from build123d import *

# Parameters (mm, degrees)
BASPROSKE_W             = 3.175
BASPROSKE_H             = 6.35
TOOTHCUT_DEPTH          = 10.525
TEETHCUTS_COUNT         = 10
TEETHCUTS_ANGLE         = 324
BORSKE_R                = 0.99949
BORE_DEPTH              = 50.8000508
SKETCH1_W               = 3.937
SKETCH1_H               = 3.937
CUT_EXTRUDE1_DEPTH      = 10.344170464
CUT_EXTRUDE1_DEPTH_BACK = 10.344170464


with BuildPart() as part:
    # BasProSke → Base-Revolve (revolve)
    with BuildSketch(Plane(origin=(0, 0, 0), x_dir=(1, 0, 0), z_dir=(0, 1, 0)), mode=Mode.PRIVATE) as base_revolve_sk:
        with Locations((1.5875, 3.175)):
            Rectangle(BASPROSKE_W, BASPROSKE_H)
    revolve(base_revolve_sk.sketch.rotate(Axis((-10, 0, 0), (1, 0, 0)), 180), axis=Axis((-10, 0, 0), (1, 0, 0)))

    # TooCutSke → ToothCut (cut, through all)
    with BuildSketch(Plane(origin=(0, 0, 0), x_dir=(0, 0, -1), z_dir=(1, 0, 0))):
        with BuildLine():
            ThreePointArc((0.630210727, 3.920537785), (0, 3.970866667), (-0.630210727, 3.920537785))
            ThreePointArc((-0.630210727, 3.920537785), (-0.900510691, 5.2110639), (-1.88228345, 6.091201374))
            ThreePointArc((-1.88228345, 6.091201374), (0, 6.3754), (1.88228345, 6.091201374))
            ThreePointArc((1.88228345, 6.091201374), (0.900510691, 5.2110639), (0.630210727, 3.920537785))
        make_face()
    toothcut = extrude(amount=TOOTHCUT_DEPTH, mode=Mode.SUBTRACT)

    # TeethCuts: ToothCut ×10 about axis
    teethcuts_axis = Axis((-10, 0, 0), (1, 0, 0))
    for i in range(1, TEETHCUTS_COUNT):
        add(toothcut.rotate(teethcuts_axis, i * TEETHCUTS_ANGLE / (TEETHCUTS_COUNT - 1)), mode=Mode.SUBTRACT)

    # BorSke → Bore (cut, symmetric)
    with BuildSketch(Plane(origin=(0, 0, 0), x_dir=(0, 0, -1), z_dir=(1, 0, 0))):
        with Locations(Location((0, 0, 0), (0, 0, 180))):
            Circle(BORSKE_R)
    extrude(amount=BORE_DEPTH, both=True, mode=Mode.SUBTRACT)

    # Sketch1 → Cut-Extrude1 (cut, two sides)
    with BuildSketch(Plane(origin=(3.175, 0, 0), x_dir=(0, 0, -1), z_dir=(1, 0, 0))) as cut_extrude1_sk:
        Rectangle(SKETCH1_W, SKETCH1_H)
    extrude(amount=CUT_EXTRUDE1_DEPTH, mode=Mode.SUBTRACT)
    extrude(cut_extrude1_sk.sketch, amount=-CUT_EXTRUDE1_DEPTH_BACK, mode=Mode.SUBTRACT)


solid = part.part
Source: CAD feature listing. Evaluate the final solid. Frame: model axes, mm. Give positions to 0.01 mm unless a question says otherwise; leave off trailing zeros. Write each loop counter-clockwise with the first axis right and the second up, starting at its lowest first coordinate (ties: lowest second). Pieces come first, ordered by that corner, then holes. Notation, with made-up numbers: M 67,62 L 97,62 A13 ccw 97,85 Z; hole C 31.5,-5 d10. An arc over 180 degrees is marked long. Return JSON: item names as keys, results as strings. Group by question number.
1) First-contact query: pin 1 Ø2 at (y, z) = (0, -4) entering from -X; pin 2 Ø1.6 at (x, z) = (2, -0.5) entering from +Y. Flat tips, straight axial feed; report the tip coordinate or a pass-through.
2) Cut plane C-C, the plane y = 3. Output: boundary loops of the cut face in (x, z) (1 decimal).
3) Cut plane D-D, the plane z = 4.25. Output: boundary loops of the cut face in (x, y) (3 decimals), then the cut area to 3 significant figures.
4) Cut plane B-B, the plane y = 5.25. Output: boundary loops of the cut face in (x, z) (3 decimals), then the cut area to 3 significant figures.
5) Cut plane A-A, the plane z = 0. Output: boundary loops of the cut face in (x, y) (1 decimal), then the cut area to 3 significant figures.
6) Draft query along Z for faces 1 (the face through (3.175, 3, 0)), 2 (the face through (1.565, -3.218, -2.327)). Return one class per face: released by +Z, released by -Z, zero draft, split by the parting line, or undercut.
7) Ray query, L1, parallel to Z at x = 1, y = 0; L2, parallel to Y at x = 1.5, z = -4.25; L3, parallel to Y at x = 1.55, z = 1.75. Return the intervals inside material, ascending.
Data:
{
 "1": {"pin 1": "stops at x = 0", "pin 2": "stops at y = 5.71"},
 "2": {"outline": "M 0,-5 L 3.2,-5 L 3.2,-2.9 L 0,-2.9 Z; M 0,-2.6 L 3.2,-2.6 L 3.2,2.6 L 0,2.6 Z; M 0,2.9 L 3.2,2.9 L 3.2,5 L 0,5 Z"},
 "3": {"outline": "M 0,-3.831 L 3.175,-3.831 L 3.175,-2.103 L 0,-2.103 Z; M 0,-0.729 L 3.175,-0.729 L 3.175,0.729 L 0,0.729 Z; M 0,2.103 L 3.175,2.103 L 3.175,3.831 L 0,3.831 Z", "area": "15.6 mm²"},
 "4": {"outline": "M 0,-2.327 L 3.175,-2.327 L 3.175,-0.924 L 0,-0.924 Z; M 0,0.924 L 3.175,0.924 L 3.175,2.327 L 0,2.327 Z", "area": "8.91 mm²"},
 "5": {"outline": "M 0,-4 L 3.2,-4 L 3.2,-2 L 0,-2 Z; M 0,2 L 3.2,2 L 3.2,4 L 0,4 Z", "area": "12.7 mm²"},
 "6": {"face 1": "zero draft", "face 2": "undercut"},
 "7": {"L1": "z = -6.35 to -1.97, 1.97 to 6.35", "L2": "y = -3.83 to -2.1, -0.73 to 0.73, 2.1 to 3.83", "L3": "y = -6.03 to -1.97, 1.97 to 6.03"}
}
